from build123d import *

# Parameters (mm, degrees)
SKETCH_1_W          = 30
SKETCH_1_H          = 10
SKETCH_1_W_2        = 26
SKETCH_1_H_2        = 6
EXTRUDE_1_DEPTH     = 77
SKETCH_2_R          = 1.5
CUT_EXTRUDE_1_DEPTH = 80.082235679


with BuildPart() as part:
    # 草图1 → 凸台-拉伸1 (new, symmetric)
    with BuildSketch(Plane(origin=(0, 0, 0), x_dir=(1, 0, 0), z_dir=(0, 1, 0))):
        Rectangle(SKETCH_1_W, SKETCH_1_H)
        Rectangle(SKETCH_1_W_2, SKETCH_1_H_2, mode=Mode.SUBTRACT)
    extrude(amount=EXTRUDE_1_DEPTH, both=True)

    # 草图2 → 切除-拉伸1 (cut, through all)
    with BuildSketch(Plane.XY.offset(5)):
        with Locations((10, 15)):
            Circle(SKETCH_2_R)
        with Locations((-10, 15)):
            Circle(SKETCH_2_R)
        with Locations((0, 15)):
            Circle(SKETCH_2_R)
        with Locations(Location((10, -15, 0), (0, 0, 180))):
            Circle(SKETCH_2_R)
        with Locations(Location((0, -15, 0), (0, 0, 180))):
            Circle(SKETCH_2_R)
        with Locations(Location((-10, -15, 0), (0, 0, 180))):
            Circle(SKETCH_2_R)
        with Locations((10, 72)):
            Circle(SKETCH_2_R)
        with Locations((-10, 72)):
            Circle(SKETCH_2_R)
        with Locations((0, 72)):
            Circle(SKETCH_2_R)
        with Locations(Location((-10, -72, 0), (0, 0, 180))):
            Circle(SKETCH_2_R)
        with Locations(Location((0, -72, 0), (0, 0, 180))):
            Circle(SKETCH_2_R)
        with Locations(Location((10, -72, 0), (0, 0, 180))):
            Circle(SKETCH_2_R)
    extrude(amount=-CUT_EXTRUDE_1_DEPTH, mode=Mode.SUBTRACT)


solid = part.part
Part model, mm, in its own coordinate system. A direction names the side the tool comes from. Coordinates: 2 decimals unless noted, no trailing zeros. Loops run counter-clockwise (first coordinate to the right, second up) from the corner with the lowest first, then second, coordinate; pieces in that order, holes last. Notation, with made-up numbers: M 69,68 L 95,68 A21 cw 95,101 Z; hole C -17,28.5 d3. An arc over 180 degrees is marked long. Use a Markdown table: item, result. Add a question column.
Q1. Cut at C-C (y = -58.5). Write the cut outline in (x, z).
Q2. Cut at A-A (y = 15). Give the number of separate pieces and of enclosed holes in the cut face, and give its area (3 significant figures).
Q3. Pin check, flat tips, straight feed: P1, Ø5, axis at x = -10, y = -72, coming from the -Z side; P2, Ø3, axis at x = -4, z = 0.5, coming from the +Y side. Stop position of each tip, or through.
Q4. Mould opens along Z. For faces 3 (the flat face through (0, 1, 5)), 4 (the flat face through (13, 1, 0)), 5 (the cylindrical face through (-11.5, 15.07, 4.01)) say: +Z half, -Z half, draft (parallel to the pull), parting line (faces both ways), or undercut.
Q5. Which spindle directions (+Z, -Z, +X, -X, +Y, -Y) get a long thin tool onto all of the face, cutting with end or side? Do faces 1 (the flat face through (0, 1, -3)), 2 (the cylindrical face through (11.5, -15.07, 4.01)). Say none if no direction does.
Q6. Cut at B-B (x = -4.5). Write the cut outline in (y, z), and give its area (3 significant figures).
Q7. Probe L1, parallel to Y at x = 10, z = -3.5; L2, parallel to X at y = 72, z = 4.4; L3, parallel to Z at x = -11.75, y = 19. List the from-to ranges inside material, lowest first.
Worked out:
| question | item | result |
|---|---|---|
| 1 | outline | M -15,-5 L 15,-5 L 15,5 L -15,5 Z; hole M -13,-3 L 13,-3 L 13,3 L -13,3 Z |
| 2 | separate pieces | 6 |
| 2 | enclosed holes | 0 |
| 2 | area | 108 mm2 |
| 3 | P1 | stops at z = -5 |
| 3 | P2 | passes through |
| 4 | face 3 | +Z half |
| 4 | face 4 | undercut |
| 4 | face 5 | draft |
| 5 | face 1 | +Y, -Y |
| 5 | face 2 | +Z, -Z |
| 6 | outline | M -77,-5 L 77,-5 L 77,-3 L -77,-3 Z; M -77,3 L 77,3 L 77,5 L -77,5 Z |
| 6 | area | 616 mm2 |
| 7 | L1 | y = -77 to -73.5, -70.5 to -16.5, -13.5 to 13.5, 16.5 to 70.5, 73.5 to 77 |
| 7 | L2 | x = -15 to -11.5, -8.5 to -1.5, 1.5 to 8.5, 11.5 to 15 |
| 7 | L3 | z = -5 to -3, 3 to 5 |
